```python
from build123d import *

# Parameters (mm, degrees)
BOSS_EXTRUDE1_DEPTH = 50
SKETCH2_R           = 3.3
CUT_EXTRUDE1_DEPTH  = 100
SKETCH3_R           = 2.5
CUT_EXTRUDE2_DEPTH  = 100
CHAMFER1_SIZE       = 0.3


with BuildPart() as part:
    # Sketch1 → Boss-Extrude1 (new, symmetric)
    with BuildSketch(Plane(origin=(0, 0, 0), x_dir=(0, 0, -1), z_dir=(1, 0, 0))):
        Polygon((0, 0), (0, 88.9), (-9.525, 88.9), (-9.525, 9.525), (-50.8, 9.525), (-50.8, 0), align=None)
    extrude(amount=BOSS_EXTRUDE1_DEPTH, both=True)

    # Sketch2 → Cut-Extrude1 (cut)
    with BuildSketch(Plane.XY.offset(9.525)):
        with Locations((-20, 77.3)):
            Circle(SKETCH2_R)
        with Locations((20, 77.3)):
            Circle(SKETCH2_R)
        with Locations((20, 24.3)):
            Circle(SKETCH2_R)
        with Locations((-20, 24.3)):
            Circle(SKETCH2_R)
    extrude(amount=-CUT_EXTRUDE1_DEPTH, mode=Mode.SUBTRACT)

    # Sketch3 → Cut-Extrude2 (cut)
    with BuildSketch(Plane(origin=(0, 9.525, 0), x_dir=(1, 0, 0), z_dir=(0, 1, 0))):
        with Locations(Location((-18, -22.025, 0), (0, 0, 270))):
            Circle(SKETCH3_R)
        with Locations(Location((-18, -44.525, 0), (0, 0, 270))):
            Circle(SKETCH3_R)
        with Locations(Location((18, -44.525, 0), (0, 0, 270))):
            Circle(SKETCH3_R)
        with Locations(Location((18, -22.025, 0), (0, 0, 270))):
            Circle(SKETCH3_R)
        with Locations(Location((0, -14.525, 0), (0, 0, 270))):
            Circle(SKETCH3_R)
    extrude(amount=-CUT_EXTRUDE2_DEPTH, mode=Mode.SUBTRACT)

    # Chamfer1
    chamfer1_edges = [part.edges().sort_by_distance(p)[0] for p in [
        (50, 88.9, 4.7625),
        (0, 0, 50.8),
        (0, 9.525, 50.8),
        (0, 9.525, 9.525),
        (0, 88.9, 9.525),
        (0, 88.9, 0),
        (0, 0, 0),
        (50, 49.2125, 9.525),
        (50, 9.525, 30.1625),
        (50, 4.7625, 50.8),
        (-23.3, 77.3, 0),
        (-23.3, 77.3, 9.525),
        (16.7, 77.3, 0),
        (16.7, 77.3, 9.525),
        (16.7, 24.3, 0),
        (16.7, 24.3, 9.525),
        (-23.3, 24.3, 0),
        (-23.3, 24.3, 9.525),
        (-18, 0, 19.525),
        (50, 0, 25.4),
        (-18, 9.525, 19.525),
        (-18, 0, 42.025),
        (-18, 9.525, 42.025),
        (18, 0, 42.025),
        (18, 9.525, 42.025),
        (18, 0, 19.525),
        (18, 9.525, 19.525),
        (0, 0, 12.025),
        (0, 9.525, 12.025),
        (-50, 4.7625, 50.8),
        (-50, 9.525, 30.1625),
        (-50, 49.2125, 9.525),
        (50, 44.45, 0),
        (-50, 88.9, 4.7625),
        (-50, 44.45, 0),
        (-50, 0, 25.4),
    ]]
    chamfer(chamfer1_edges, length=CHAMFER1_SIZE)


solid = part.part
```
For this review, take the finished solid that the model builds, in its own axes (mm). A direction names the side the tool comes from. Round coordinates to 2 decimals unless told otherwise and drop trailing zeros. Write each loop counter-clockwise with the first axis right and the second up, starting at its lowest first coordinate (ties: lowest second). Pieces come first, ordered by that corner, then holes.
1) Take a section at A-A on y = 24.3. Give the boundary of the cut face in (x, z) (3 decimals).
Answer below:
outline: (-50, 0.3) - (-49.7, 0) - (-23.6, 0) - (-23.3, 0.3) - (-23.3, 9.225) - (-23.6, 9.525) - (-49.7, 9.525) - (-50, 9.225) - close; (-16.7, 0.3) - (-16.4, 0) - (16.4, 0) - (16.7, 0.3) - (16.7, 9.225) - (16.4, 9.525) - (-16.4, 9.525) - (-16.7, 9.225) - close; (23.3, 0.3) - (23.6, 0) - (49.7, 0) - (50, 0.3) - (50, 9.225) - (49.7, 9.525) - (23.6, 9.525) - (23.3, 9.225) - close
2) Insertion check: pin 1 Ø6 at (x, y) = (-20, 24.3) entering from -Z; pin 2 Ø6.5 at (x, z) = (18, 22.025) entering from +Y (3 decimals); pin 3 Ø23.5 at (x, y) = (-22.5, 36.5) entering from +Z (3 decimals). Each pin has a flat end and moves straight along its axis. Give the tip position at first contact, or say it passes through.
Answer below:
pin 1: passes through
pin 2: stops at y = 9.525
pin 3: stops at z = 9.525
3) For line 1 along Y through (x, z) = (20, 2); line 2 along Y through (x, z) = (-17, 17) (3 decimals), list the stretches that pass through material, from the lowest coordinate up.
Answer below:
line 1: y = 0 to 21, 27.6 to 74, 80.6 to 88.9
line 2: y = 0 to 9.525
4) Take a section at D-D on y = 63. Give the boundary of the cut face in (x, z) (3 decimals), then the cut area to 3 significant figures.
Answer below:
outline: (-50, 0.3) - (-49.7, 0) - (49.7, 0) - (50, 0.3) - (50, 9.225) - (49.7, 9.525) - (-49.7, 9.525) - (-50, 9.225) - close
area: 952 mm2
5) Take a section at B-B on x = 0. Give the boundary of the cut face in (y, z) (3 decimals), then the cut area to 3 significant figures.
Answer below:
outline: (0, 0.3) - (0.3, 0) - (88.6, 0) - (88.9, 0.3) - (88.9, 9.225) - (88.6, 9.525) - (9.825, 9.525) - (9.525, 9.825) - (9.525, 11.725) - (9.225, 12.025) - (0.3, 12.025) - (0, 11.725) - close; (0, 17.325) - (0.3, 17.025) - (9.225, 17.025) - (9.525, 17.325) - (9.525, 50.5) - (9.225, 50.8) - (0.3, 50.8) - (0, 50.5) - close
area: 1,190 mm2
6) Take a section at C-C on y = 8. Give the boundary of the cut face in (x, z) (3 decimals).
Answer below:
outline: (-50, 0.3) - (-49.7, 0) - (49.7, 0) - (50, 0.3) - (50, 50.5) - (49.7, 50.8) - (-49.7, 50.8) - (-50, 50.5) - close; hole circle Ø5 at (-18, 22.025); hole circle Ø5 at (-18, 44.525); hole circle Ø5 at (0, 14.525); hole circle Ø5 at (18, 22.025); hole circle Ø5 at (18, 44.525)
7) Machinability: for faces 1 (the face through (1, 9.525, 30)), 2 (the face through (1, 5, 50.8)), which of the approach directions +Z, -Z, +X, -X, +Y, -Y give a long, thin tool a straight path to every point of the face, cutting with its end or side? Answer none if there is none.
Answer below:
face 1: +Z, +X, -X, +Y
face 2: +Z, +X, -X, +Y, -Y
8) Mouldability with a two-part tool opening along Z and no side actions: class faces 3 (the face through (-16.95, 23.04, 4.82)), 4 (the face through (18.75, 4.82, 46.91)), 5 (the face through (1, 50, 9.525)) as +Z half, -Z half, draft (parallel to the pull), parting line (faces both ways), or undercut.
Answer below:
face 3: draft
face 4: undercut
face 5: +Z half
